Build history of the part. All positions in model axes, mm. A direction names the side the tool comes from. Coordinates: 2 decimals unless noted, no trailing zeros. Order: outer loops, then holes, each group sorted by start corner. A loop starts at its lowest first (then second) coordinate and runs counter-clockwise, first axis right, second up. Notation, with made-up numbers: (-24.5, 17) - (0.5, 17) arc R20 cw to (0.5, 37) - close; hole circle Ø9 at (-16, 72). An arc over 180 degrees is marked (long way). One line per item, written item: value.
from build123d import *

# Parameters (mm, degrees)
F0_W     = 44
F0_H     = 59
F0_W_2   = 30
F0_H_2   = 22
F1_DEPTH = 10
F2_W     = 30
F2_H     = 3
F3_DEPTH = 3
F4_W     = 38
F4_H     = 3
F5_DEPTH = 2
F6_W     = 3
F6_H     = 15
F6_W_2   = 2
F7_DEPTH = 24
F8_DEPTH = 10
F9_R     = 1.99999


# Not quite as in the source:
# - a fillet or chamfer is up to 0.001 mm smaller than in the source, because OpenCascade refuses the exact size


with BuildPart() as f1:
    # F0 (on Top) → F1 (new body)
    with BuildSketch(Plane.XY):
        with Locations((0, -11)):
            Rectangle(F0_W, F0_H)
        with Locations((0, -1)):
            Rectangle(F0_W_2, F0_H_2, mode=Mode.SUBTRACT)
    extrude(amount=F1_DEPTH)

    # F2 (on face) → F3 (cut)
    with BuildSketch(Plane.XY.offset(10)):
        with Locations((0, -13.5)):
            Rectangle(F2_W, F2_H)
        with Locations((0, 11.5)):
            Rectangle(F2_W, F2_H)
    extrude(amount=-F3_DEPTH, mode=Mode.SUBTRACT)

    # F4 (on face) → F5 (join)
    with BuildSketch(Plane.XY.offset(10)):
        with Locations((0, 17)):
            Rectangle(F4_W, F4_H)
    extrude(amount=F5_DEPTH)

    # F6 (on face) → F7 (join)
    with BuildSketch(Plane.XY.offset(10)):
        with Locations((-20.5, 5)):
            Rectangle(F6_W, F6_H)
        with Locations((-23, 5)):
            Rectangle(F6_W_2, F6_H)
        with Locations((-23, -30)):
            Rectangle(F6_W_2, F6_H)
        with Locations((-20.5, -30)):
            Rectangle(F6_W, F6_H)
        with Locations((23, 5)):
            Rectangle(F6_W_2, F6_H)
        with Locations((23, -30)):
            Rectangle(F6_W_2, F6_H)
        with Locations((20.5, -30)):
            Rectangle(F6_W, F6_H)
        with Locations((20.5, 5)):
            Rectangle(F6_W, F6_H)
    extrude(amount=F7_DEPTH)

    # F6 (on face) → F8 (join, through all)
    with BuildSketch(Plane.XY.offset(10)):
        with Locations((-23, -30)):
            Rectangle(F6_W_2, F6_H)
        with Locations((-23, 5)):
            Rectangle(F6_W_2, F6_H)
        with Locations((23, -30)):
            Rectangle(F6_W_2, F6_H)
        with Locations((23, 5)):
            Rectangle(F6_W_2, F6_H)
    extrude(amount=-F8_DEPTH)

    # F9 (radius 2 in the source; OpenCascade refuses exactly that, so slightly less here)
    f9_edges = [f1.edges().sort_by_distance(p)[0] for p in [
        (24, 12.5, 17),
        (-24, 12.5, 17),
        (-24, -2.5, 17),
        (-24, -22.5, 17),
        (-24, -37.5, 17),
        (24, -37.5, 17),
        (24, -22.5, 17),
        (22, -40.5, 5),
        (-22, -40.5, 5),
        (22, 18.5, 5),
        (-22, 18.5, 5),
        (24, -2.5, 17),
        (-15, 13, 8.5),
        (15, 13, 8.5),
        (-15, -15, 8.5),
        (15, -15, 8.5),
    ]]
    fillet(f9_edges, radius=F9_R)


solid = f1.part
1. Band-saw the part on D-D, the plane y = -11. Give the cut face in (x, z), and give its area (3 significant figures).
Values found:
outline: (-22, 0) - (-15, 0) - (-15, 10) - (-22, 10) - close; (15, 0) - (22, 0) - (22, 10) - (15, 10) - close
area: 140 mm2
2. 3-axis set-ups, long thin cutter, end or side, ignore diameter. For faces 4 (the face through (22, -13, 5)), 5 (the face through (0, 15.5, 11)), 6 (the face through (14.43, 12.4, 8.48)), 7 (the face through (-22, 14, 5)): which of +Z, -Z, +X, -X, +Y, -Y reach the whole face in a straight line?
Values found:
face 4: +Z, -Z, +X
face 5: +Z, +X, -X, -Y
face 6: +Z
face 7: +Z, -Z, -X, +Y
3. Flat gauge pins, fed straight in: P1, Ø0.5, axis at y = -38, z = 4.5, coming from the -X side; P2, Ø2, axis at y = 17, z = 11.5, coming from the -X side; P3, Ø8, axis at y = -9, z = 28.5, coming from the +X side; P4, Ø1.5, axis at x = 21, z = 17, coming from the +Y side. Where does each tip first touch, or does it go through?
Values found:
P1: stops at x = -22
P2: stops at x = -19
P3: passes through
P4: stops at y = 12.5
4. Two-plate mould, pull along Y, no slides. Class faces 1 (the face through (21, -30, 34)), 2 (the face through (21.4, -39.93, 5.07)), 3 (the face through (0, -13, 7)): pulls with the +Y half, pulls with the -Y half, needs draft (parallel to the pull), parting line crosses it, or undercut.
Values found:
face 1: needs draft
face 2: pulls with the -Y half
face 3: undercut
5. Band-saw the part on C-C, the plane y = 7. Give the cut face in (x, z).
Values found:
outline: (-24, 0) - (-15, 0) - (-15, 10) - (-19, 10) - (-19, 34) - (-24, 34) - close; (15, 0) - (24, 0) - (24, 34) - (19, 34) - (19, 10) - (15, 10) - close
6. Band-saw the part on B-B, the plane z = 29. Give the cut face in (x, y).
Values found:
outline: (-24, -35.5) arc R2 ccw to (-22, -37.5) - (-19, -37.5) - (-19, -22.5) - (-22, -22.5) arc R2 ccw to (-24, -24.5) - close; (-24, -0.5) arc R2 ccw to (-22, -2.5) - (-19, -2.5) - (-19, 12.5) - (-22, 12.5) arc R2 ccw to (-24, 10.5) - close; (19, -37.5) - (22, -37.5) arc R2 ccw to (24, -35.5) - (24, -24.5) arc R2 ccw to (22, -22.5) - (19, -22.5) - close; (19, -2.5) - (22, -2.5) arc R2 ccw to (24, -0.5) - (24, 10.5) arc R2 ccw to (22, 12.5) - (19, 12.5) - close
7. Band-saw the part on A-A, the plane x = -11. Give the cut face in (y, z).
Values found:
outline: (-40.5, 0) - (-12, 0) - (-12, 7) - (-15, 7) - (-15, 10) - (-40.5, 10) - close; (10, 0) - (18.5, 0) - (18.5, 12) - (15.5, 12) - (15.5, 10) - (13, 10) - (13, 7) - (10, 7) - close
8. Probe line 1 along Y through (x, z) = (-3, 7.5); line 2 along X through (y, z) = (0.5, 16); line 3 along X through (y, z) = (-6, 5). List the from-to ranges inside material, lowest first.
Values found:
line 1: y = -40.5 to -15, 13 to 18.5
line 2: x = -24 to -19, 19 to 24
line 3: x = -22 to -15, 15 to 22
